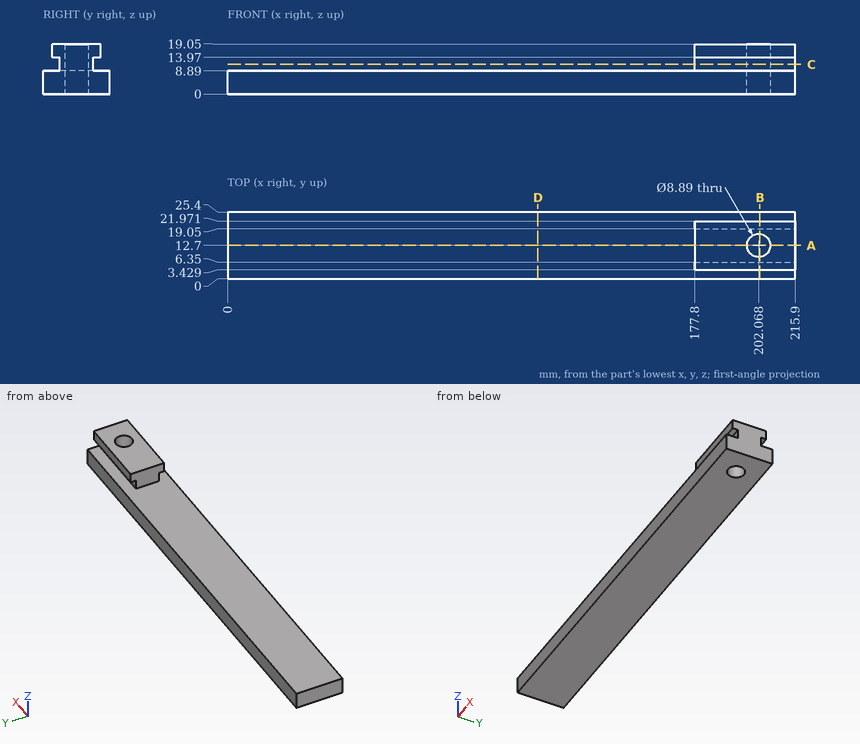
Check sheet for the drawn part. Datum: minimum x, y, z corner. Units: mm. Round coordinates to 2 decimals unless told otherwise and drop trailing zeros. Order: outer loops, then holes, each group sorted by start corner. A loop starts at its lowest first (then second) coordinate and runs counter-clockwise, first axis right, second up.
1. Thickness scan on L1, parallel to X at y = 13.25, z = 9.75; L2, parallel to Z at x = 95.5, y = 11; L3, parallel to X at y = 7.75, z = 14.75. Record the ranges inside material, lowest first.
Final values:
L1: x = 177.8 to 197.66, 206.48 to 215.9
L2: z = 0 to 8.89
L3: x = 177.8 to 215.9
2. Section check D-D on x = 118. Record the cut outline in (y, z).
Final values:
outline: (0, 0) - (25.4, 0) - (25.4, 8.89) - (0, 8.89) - close
3. Section check C-C on z = 11.25. Record the cut outline in (x, y) (3 decimals).
Final values:
outline: (177.8, 6.35) - (215.9, 6.35) - (215.9, 19.05) - (177.8, 19.05) - close; hole circle Ø8.89 at (202.068, 12.7)
4. Section check B-B on x = 202.5. Record the cut outline in (y, z), then the cut area to 3 significant figures.
Final values:
outline: (0, 0) - (8.28, 0) - (8.28, 19.05) - (3.43, 19.05) - (3.43, 13.97) - (6.35, 13.97) - (6.35, 8.89) - (0, 8.89) - close; (17.12, 0) - (25.4, 0) - (25.4, 8.89) - (19.05, 8.89) - (19.05, 13.97) - (21.97, 13.97) - (21.97, 19.05) - (17.12, 19.05) - close
area: 216 mm2
5. Section check A-A on y = 12.7. Record the cut outline in (x, z).
Final values:
outline: (0, 0) - (197.62, 0) - (197.62, 19.05) - (177.8, 19.05) - (177.8, 8.89) - (0, 8.89) - close; (206.51, 0) - (215.9, 0) - (215.9, 19.05) - (206.51, 19.05) - close
6. Go/stop test with flat-tipped pins: P1, Ø5.5, axis at x = 194.5, z = 12.5, coming from the -Y side; P2, Ø12.5, axis at x = 62.5, y = 14.5, coming from the +Z side; P3, Ø1.5, axis at x = 201, z = 15.5, coming from the +Y side. Record where each tip stops, or that it passes through.
Final values:
P1: stops at y = 3.43
P2: stops at z = 8.89
P3: stops at y = 21.97
